from build123d import *

# Parameters (mm, degrees)
F0_W     = 25.4
F0_H     = 76.2
F1_DEPTH = 127
F3_DEPTH = 177.8
F4_W     = 24.25904
F4_H     = 7.62
F5_DEPTH = 25.4


with BuildPart() as f1:
    # F0 (on Front) → F1 (new body)
    with BuildSketch(Plane.XZ):
        Rectangle(F0_W, F0_H)
    extrude(amount=F1_DEPTH)

    # F2 (on face) → F3 (cut)
    with BuildSketch(Plane.XZ.offset(127)):
        Polygon((6.35, 26.099518), (12.7, 26.099518), (12.7, 38.1), (-12.7, 38.1), (-12.7, 26.099518), (-6.35, 26.099518), (-6.35, 33.719518), (6.35, 33.719518), align=None)
    extrude(amount=-F3_DEPTH, mode=Mode.SUBTRACT)

    # F4 (on face) → F5 (cut)
    with BuildSketch(Plane.YZ.offset(6.35)):
        Polygon((-100.70353, 29.807648), (-84.444813, 33.719518), (-127, 33.719518), (-127, 26.099518), (-105.267383, 26.099518), align=None)
        with Locations((-12.12952, 29.909518)):
            Rectangle(F4_W, F4_H)
    extrude(amount=-F5_DEPTH, mode=Mode.SUBTRACT)


solid = f1.part
CAD build for the part. Positions are in the model's coordinates, mm. A direction names the side the tool comes from. Give positions to 0.01 mm unless a question says otherwise; leave off trailing zeros. Write each loop counter-clockwise with the first axis right and the second up, starting at its lowest first coordinate (ties: lowest second). Pieces come first, ordered by that corner, then holes. Notation, with made-up numbers: (4, 87.5) - (58, 87.5) arc R22 cw to (58, 103.5) - close; hole circle Ø11 at (88.5, 58.5). An arc over 180 degrees is marked (long way). Answer as CSV lines item,"result".
Q1. Band-saw the part on A-A (x = 1.5). Give the cut face in (y, z), and give its area (3 significant figures).
Result set:
outline,"(-127, -38.1) - (0, -38.1) - (0, 26.1) - (-24.26, 26.1) - (-24.26, 33.72) - (-84.44, 33.72) - (-100.7, 29.81) - (-105.27, 26.1) - (-127, 26.1) - close"
area,"8,710 mm²"
Q2. Band-saw the part on D-D (x = -9). Give the cut face in (y, z).
Result set:
outline,"(-127, -38.1) - (0, -38.1) - (0, 26.1) - (-127, 26.1) - close"
Q3. 3-axis set-ups, long thin cutter, end or side, ignore diameter. For faces 1 (the face through (6.35, -65, 30)), 2 (the face through (0, -127, -6)), 3 (the face through (-6.35, -65, 30)), 4 (the face through (0, -24.259, 30)), 5 (the face through (0, -55, 33.72)): which of +Z, -Z, +X, -X, +Y, -Y reach the whole face in a straight line?
Result set:
face 1,"+Z, +X, +Y, -Y"
face 2,"+Z, -Z, +X, -X, -Y"
face 3,"+Z, -X, +Y, -Y"
face 4,"+Z, +X, -X, +Y"
face 5,"+Z, +X, -X, +Y, -Y"
Q4. Band-saw the part on C-C (z = 28.5). Give the cut face in (x, y).
Result set:
outline,"(-6.35, -102.31) - (6.35, -102.31) - (6.35, -24.26) - (-6.35, -24.26) - close"
Q5. Drill centre lines: line 1 (Z direction, x = -9.25, y = -6.5); line 2 (Y direction, x = 3.75, z = 28). Where is each one in solid material? Low to high. Write a range as from..to.
Result set:
line 1,"-38.1..26.1"
line 2,"-102.93..-24.26"
Q6. Band-saw the part on B-B (y = -62). Give the cut face in (x, z).
Result set:
outline,"(-12.7, -38.1) - (12.7, -38.1) - (12.7, 26.1) - (6.35, 26.1) - (6.35, 33.72) - (-6.35, 33.72) - (-6.35, 26.1) - (-12.7, 26.1) - close"
Q7. Flat gauge pins, fed straight in: pin 1 Ø3 at (x, y) = (9.5, -101) entering from +Z; pin 2 Ø4 at (y, z) = (-83, 31) entering from +X; pin 3 Ø4 at (x, z) = (-3, 30) entering from +Y. Where does each tip first touch, or does it go through?
Result set:
pin 1,"z = 26.1"
pin 2,"x = 6.35"
pin 3,"y = -24.26"
